Here's how the part is built. I have some questions about the finished solid (model axes, mm). Face numbers are marked on the shaded views. A direction names the side the tool comes from. Coordinates: 2 decimals unless noted, no trailing zeros. Loops run counter-clockwise (first coordinate to the right, second up) from the corner with the lowest first, then second, coordinate; pieces in that order, holes last. Notation, with made-up numbers: M 77.5,36.25 L 101.5,36.25 A13 ccw 101.5,41.25 Z; hole C 47,78 d5. An arc over 180 degrees is marked long. Use CSV: the item, a comma, the result in double quotes. Start each with the question number.
Q1. For pin 1 Ø11.5 at (x, y) = (-76.2, 0) entering from +Z; pin 2 Ø10 at (y, z) = (11.5, 49.5) entering from +X; pin 3 Ø8 at (x, z) = (73.5, 59.5) entering from -Y; pin 4 Ø6 at (x, z) = (28.5, 26.5) entering from -Y, each with a flat end and sliding along its axis, tell me the tip position at first contact or that it passes through.
Q2. Which directions (+Z, -Z, +X, -X, +Y, -Y) give clear straight access to the entire face, cutting with the end or side of a thin tool? Please do the marked faces 1 and 2.
Q3. If we section it at C-C (z = 48.5): Please give me the cut outline in (x, y).
Q4. If we section it at A-A (x = -76.2): Please give me the cut outline in (y, z).
Q5. Please list where these lines run through material, in increasing order: probe 1 along Y at (x, z) = (0, 54); probe 2 along Z at (x, y) = (41.5, 64); probe 3 along Y at (x, z) = (33.5, 30.5). Write a range as [from, to].
Q6. If we mould it in two halves opening along Y, with no side actions, what happens to the marked faces 3, 4, 5 and 6? For each: +Y half, -Y half, draft (parallel to the pull), parting line (faces both ways), or undercut.
Q7. If we section it at D-D (y = 0): Please give me the cut outline in (x, z), and give its area (3 significant figures).
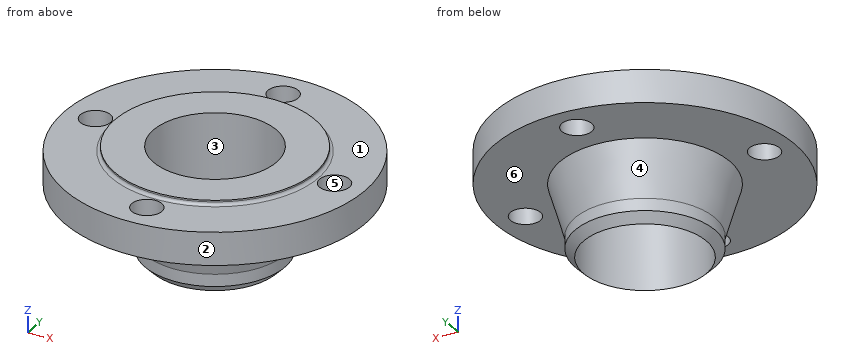
from build123d import *

# Parameters (mm, degrees)
F2_R     = 9.55
F3_DEPTH = 66.901


with BuildPart() as f1:
    # F0 (on Front) → F1 (revolve)
    with BuildSketch(Plane.XZ):
        with BuildLine():
            Line((-44.45, 5.45), (-39, 0))
            Line((-39, 0), (-39, 69.9))
            Line((-39, 69.9), (-63.5, 69.9))
            Line((-63.5, 69.9), (-63.5, 68.9))
            ThreePointArc((-63.5, 68.9), (-64.085786, 67.485786), (-65.5, 66.9))
            Line((-65.5, 66.9), (-95.25, 66.9))
            Line((-95.25, 66.9), (-95.25, 46))
            Line((-95.25, 46), (-54, 46))
            Line((-54, 46), (-44.45, 13.157464))
            Line((-44.45, 13.157464), (-44.45, 5.45))
        make_face()
    revolve(axis=Axis((0, 0, 36.061939), (0, 0, 1)))

    # F2 (on face) → F3 (cut, through all)
    with BuildSketch(Plane.XY.offset(66.9)):
        with Locations((-76.2, 0)):
            Circle(F2_R)
        with Locations((0, -76.2)):
            Circle(F2_R)
        with Locations((76.2, 0)):
            Circle(F2_R)
        with Locations((0, 76.2)):
            Circle(F2_R)
    extrude(amount=-F3_DEPTH, mode=Mode.SUBTRACT)


solid = f1.part
Results below:
1,pin 1,"through"
1,pin 2,"x = 95.03"
1,pin 3,"y = -65.13"
1,pin 4,"y = -41.32"
2,face 1,"+Z"
2,face 2,"+Z, -Z"
3,outline,"C 0,0 d190.5; hole C -76.2,0 d19.1; hole C 0,0 d78; hole C 0,-76.2 d19.1; hole C 0,76.2 d19.1; hole C 76.2,0 d19.1"
4,outline,"M -57.15,46 L -9.55,46 L -9.55,66.9 L -57.15,66.9 Z; M 9.55,46 L 57.15,46 L 57.15,66.9 L 9.55,66.9 Z"
5,probe 1,"[-95.25, -85.75], [-66.65, -39], [39, 66.65], [85.75, 95.25]"
5,probe 2,"[46, 66.9]"
5,probe 3,"[-36.43, -19.97], [19.97, 36.43]"
6,face 3,"undercut"
6,face 4,"parting line"
6,face 5,"undercut"
6,face 6,"draft"
7,outline,"M -95.25,46 L -85.75,46 L -85.75,66.9 L -95.25,66.9 Z; M -66.65,46 L -54,46 L -44.45,13.16 L -44.45,5.45 L -39,0 L -39,69.9 L -63.5,69.9 L -63.5,68.9 A2 cw -65.5,66.9 L -66.65,66.9 Z; M 39,0 L 44.45,5.45 L 44.45,13.16 L 54,46 L 66.65,46 L 66.65,66.9 L 65.5,66.9 A2 cw 63.5,68.9 L 63.5,69.9 L 39,69.9 Z; M 85.75,46 L 95.25,46 L 95.25,66.9 L 85.75,66.9 Z"
7,area,"2,490 mm^2"
